Design review of the part shown in the three views and the two pictorial views. Dimensions are in mm from the part's minimum x, y and z. A direction names the side the tool comes from. Round coordinates to 2 decimals unless told otherwise and drop trailing zeros. Order: outer loops, then holes, each group sorted by start corner. A loop starts at its lowest first (then second) coordinate and runs counter-clockwise, first axis right, second up. Notation, with made-up numbers: M 66.25,52.25 L 113.25,52.25 A7 ccw 113.25,58.25 Z; hole C -36.5,-21 d5. An arc over 180 degrees is marked long. Write each question's results on one line, items separated by ' | '. Start each with the question number.
Item 1: Take a section at B-B, the plane y = 7. Write out the cut boundary in (x, z), plus the area to 3 significant figures.
Item 2: Machinability: for the marked faces 1 and 2, which of the approach directions +Z, -Z, +X, -X, +Y, -Y give a long, thin tool a straight path to every point of the face, cutting with its end or side? Answer none if there is none.
Item 3: Wall thickness on line 1 (Z direction, x = 8, y = 23.5); line 2 (Z direction, x = 17.5, y = 40); line 3 (Y direction, x = 17, z = 27): over which ranges is each line inside the solid? List them lowest first. Write a range as [from, to].
Item 4: Take a section at A-A, the plane x = 12.25. Write out the cut boundary in (y, z) (3 decimals), plus the area to 3 significant figures.
Item 5: Clearance check with a flat-ended pin moving along its axis: pin 1 (6 mm diameter, centred on x = 15.5, y = 13.5, fed in from +Z). State where the tip first meets the part, or that it passes through.
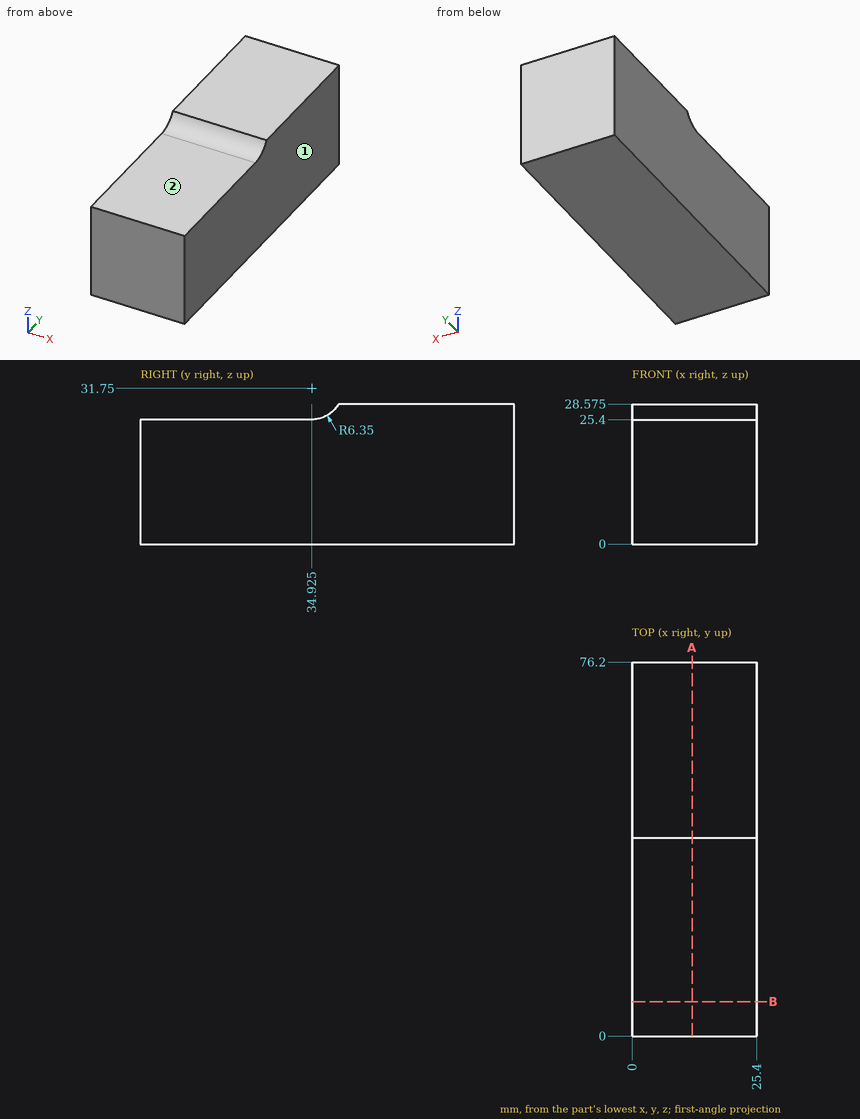
Results list:
1) outline: M 0,0 L 25.4,0 L 25.4,25.4 L 0,25.4 Z | area: 645 mm²
2) face 1: +Z, -Z, +X, +Y, -Y | face 2: +Z, +X, -X, -Y
3) line 1: [0, 25.4] | line 2: [0, 27.93] | line 3: [39.14, 76.2]
4) outline: M 0,0 L 76.2,0 L 76.2,28.575 L 40.424,28.575 A6.35 cw 34.925,25.4 L 0,25.4 Z | area: 2,050 mm²
5) pin 1: z = 25.4
